Can you work these out from the model? Positions are in its coordinate system, mm. A direction names the side the tool comes from. Coordinates: 2 decimals unless noted, no trailing zeros. Order: outer loops, then holes, each group sorted by start corner. A loop starts at its lowest first (then second) coordinate and runs counter-clockwise, first axis right, second up. Notation, with made-up numbers: (62, 71) - (107, 71) arc R26 ccw to (107, 95) - close; hole circle Ø1 at (43, 50). An arc over 180 degrees is marked (long way). Use a Markdown table: item, result. Add a question column.
(1) For pin 1 Ø2.5 at (x, z) = (-75.4, -19.55) entering from -Y; pin 2 Ø1 at (x, y) = (-82.5, 2) entering from +Z; pin 3 Ø0.6 at (y, z) = (1.5, 64.5) entering from -X; pin 4 Ø1.7 at (y, z) = (1.5, -64) entering from -X, each with a flat end and sliding along its axis, tell me the tip position at first contact or that it passes through.
(2) I want a section at A-A (x = 55). List the corners of the cut face in (y, z) for me, and give its area (3 significant figures).
(3) I want a section at B-B (y = 0.65). State how many separate pieces and enclosed holes the cut face has, and give its area (3 significant figures).
(4) If I drill on L1, parallel to Z at x = -67, y = 2.35; L2, parallel to Z at x = 55, y = 2; L3, parallel to X at y = 1.1, z = 37 (3 decimals), over which ranges is the centre line in solid material (lowest first)? Write a range as [from, to].
(5) We'd pull the mould along Z, two halves only. Please class faces 1 (the cylindrical face through (-77.5, 1.48, 19.33)), 2 (the cylindrical face through (-44.031, 1.479, -58.137)), 3 (the flat face through (-34, 0, -1)), 4 (the cylindrical face through (-134.983, 1.479, 1.539)): pulls with the +Z half, pulls with the -Z half, needs draft (parallel to the pull), parting line crosses it, or undercut.
(6) On a 3-axis mill with a long thin cutter (end or side, diameter ignored), from which of +Z, -Z, +X, -X, +Y, -Y can I reach the whole of each face in a straight line? I mean faces 5 (the flat face through (-34, 3, -1)), 6 (the cylindrical face through (-129.984, 1.479, 1.429)). Say none if no direction works.
(7) I want a section at C-C (x = -112). List the corners of the cut face in (y, z) for me, and give its area (3 significant figures).
```python
from build123d import *

# Parameters (mm, degrees)
SKETCH1_R           = 2.1
SKETCH1_R_2         = 1.5
SKETCH1_R_3         = 2
SKETCH1_R_4         = 3
BOSS_EXTRUDE1_DEPTH = 3


with BuildPart() as part:
    # Sketch1 → Boss-Extrude1 (new body)
    with BuildSketch(Plane(origin=(0, 0, 0), x_dir=(1, 0, 0), z_dir=(0, 1, 0))):
        with BuildLine():
            Line((65, -70), (-65, -70))
            ThreePointArc((-65, -70), (-135, 0), (-65, 70))
            Line((-65, 70), (65, 70))
            Line((65, 70), (65, -70))
        make_face()
        with Locations((-45, -60)):
            Circle(SKETCH1_R, mode=Mode.SUBTRACT)
        with Locations((-45, 60)):
            Circle(SKETCH1_R, mode=Mode.SUBTRACT)
        with Locations((55, -60)):
            Circle(SKETCH1_R, mode=Mode.SUBTRACT)
        with Locations((55, 60)):
            Circle(SKETCH1_R, mode=Mode.SUBTRACT)
        with Locations((37.841964001, -25.6)):
            Circle(SKETCH1_R_2, mode=Mode.SUBTRACT)
        with Locations((37.841964001, -56.6)):
            Circle(SKETCH1_R_2, mode=Mode.SUBTRACT)
        with Locations((38.099271459, 44.2)):
            Circle(SKETCH1_R_2, mode=Mode.SUBTRACT)
        with Locations((38.099271459, 62.8)):
            Circle(SKETCH1_R_2, mode=Mode.SUBTRACT)
        with Locations((-75.400632029, -19.426149967)):
            Circle(SKETCH1_R, mode=Mode.SUBTRACT)
        with Locations((-75.399684811, 19.552626294)):
            Circle(SKETCH1_R_3, mode=Mode.SUBTRACT)
        with Locations((-105.935731265, 33.388623858)):
            Circle(SKETCH1_R_4, mode=Mode.SUBTRACT)
        with Locations((-105.935731265, -35.611376142)):
            Circle(SKETCH1_R_4, mode=Mode.SUBTRACT)
        with BuildLine():
            Line((-65, 65), (-65, 62.9))
            ThreePointArc((-65, 62.9), (-127.9, 0), (-65, -62.9))
            Line((-65, -62.9), (-65, -65))
            ThreePointArc((-65, -65), (-130, 0), (-65, 65))
        make_face(mode=Mode.SUBTRACT)
    extrude(amount=BOSS_EXTRUDE1_DEPTH)


solid = part.part
```
Answers follow:
| question | item | result |
|---|---|---|
| 1 | pin 1 | passes through |
| 1 | pin 2 | stops at z = 67.9 |
| 1 | pin 3 | stops at x = -92.9 |
| 1 | pin 4 | stops at x = -95.2 |
| 2 | outline | (0, -70) - (3, -70) - (3, -62.1) - (0, -62.1) - close; (0, -57.9) - (3, -57.9) - (3, 57.9) - (0, 57.9) - close; (0, 62.1) - (3, 62.1) - (3, 70) - (0, 70) - close |
| 2 | area | 395 mm² |
| 3 | separate pieces | 1 |
| 3 | enclosed holes | 13 |
| 3 | area | 25,300 mm² |
| 4 | L1 | z = [-69.97, -64.97], [-62.87, 62.87], [64.97, 69.97] |
| 4 | L2 | z = [-70, -62.1], [-57.9, 57.9], [62.1, 70] |
| 4 | L3 | x = [-124.422, -118.442], [-115.867, -108.595], [-103.276, 65] |
| 5 | face 1 | undercut |
| 5 | face 2 | undercut |
| 5 | face 3 | needs draft |
| 5 | face 4 | parting line crosses it |
| 6 | face 5 | +Z, -Z, +X, -X, +Y |
| 6 | face 6 | +Y, -Y |
| 7 | outline | (0, -51.87) - (3, -51.87) - (3, -44.9) - (0, -44.9) - close; (0, -41.8) - (3, -41.8) - (3, 41.8) - (0, 41.8) - close; (0, 44.9) - (3, 44.9) - (3, 51.87) - (0, 51.87) - close |
| 7 | area | 293 mm² |
